```python
from build123d import *

# Parameters (mm, degrees)
BOSS_EXTRUDE1_DEPTH          = 1.5
SKETCH1_3_W                  = 3.18
SKETCH1_3_H                  = 20
CUT_EXTRUDE_THIN1_DEPTH      = 2.5
CUT_EXTRUDE_THIN1_DEPTH_BACK = 2.5
CUT_EXTRUDE1_REACH           = 5


with BuildPart() as part:
    # Sketch1 → Boss-Extrude1 (new body, symmetric)
    with BuildSketch(Plane.XY):
        Polygon((-93.914893617, 114.397705985), (-93.914893617, -65.602294015), (86.085106383, -65.602294015), (86.085106383, -25.602294015), (-3.914893617, -25.602294015), (-3.914893617, 84.397705985), (-33.914893617, 114.397705985), align=None)
    extrude(amount=BOSS_EXTRUDE1_DEPTH, both=True)

    # Sketch1_3 → Cut-Extrude-Thin1 (cut, two sides)
    with BuildSketch(Plane.XY) as cut_extrude_thin1_sk:
        with Locations((-92.414893617, 64.397705985)):
            Rectangle(SKETCH1_3_W, SKETCH1_3_H)
        with Locations((-92.414893617, 24.397705985)):
            Rectangle(SKETCH1_3_W, SKETCH1_3_H)
        with Locations((-92.414893617, -15.602294015)):
            Rectangle(SKETCH1_3_W, SKETCH1_3_H)
        with Locations((-5.414893617, 54.397705985)):
            Rectangle(SKETCH1_3_W, SKETCH1_3_H)
        with Locations((-5.414893617, 4.397705985)):
            Rectangle(SKETCH1_3_W, SKETCH1_3_H)
        with Locations((84.585106383, -45.602294015)):
            Rectangle(SKETCH1_3_W, SKETCH1_3_H)
    extrude(amount=CUT_EXTRUDE_THIN1_DEPTH, mode=Mode.SUBTRACT)
    extrude(cut_extrude_thin1_sk.sketch, amount=-CUT_EXTRUDE_THIN1_DEPTH_BACK, mode=Mode.SUBTRACT)

    # Sketch2 → Cut-Extrude1 (cut, up to next)
    with BuildSketch(Plane.XY.offset(1.5), mode=Mode.PRIVATE) as cut_extrude1_sk1:
        Polygon((-25.473348524, -46.697563546), (-7.347192784, -55.14992878), (-6.079337999, -52.431005419), (-24.205493739, -43.978640185), align=None)
    cut_extrude1_tool1 = extrude(cut_extrude1_sk1.sketch, amount=-CUT_EXTRUDE1_REACH, mode=Mode.PRIVATE) & part.part
    add(cut_extrude1_tool1.solids().sort_by_distance((-15.776343, -49.564284, 1.5))[0], mode=Mode.SUBTRACT)
    # Sketch2 → Cut-Extrude1 (cut, up to next)
    with BuildSketch(Plane.XY.offset(1.5), mode=Mode.PRIVATE) as cut_extrude1_sk2:
        Polygon((-51.39472735, -31.300092332), (-69.520883091, -22.847727097), (-70.788737876, -25.566650459), (-52.662582136, -34.019015693), align=None)
    cut_extrude1_tool2 = extrude(cut_extrude1_sk2.sketch, amount=-CUT_EXTRUDE1_REACH, mode=Mode.PRIVATE) & part.part
    add(cut_extrude1_tool2.solids().sort_by_distance((-61.091733, -28.433371, 1.5))[0], mode=Mode.SUBTRACT)


solid = part.part
```
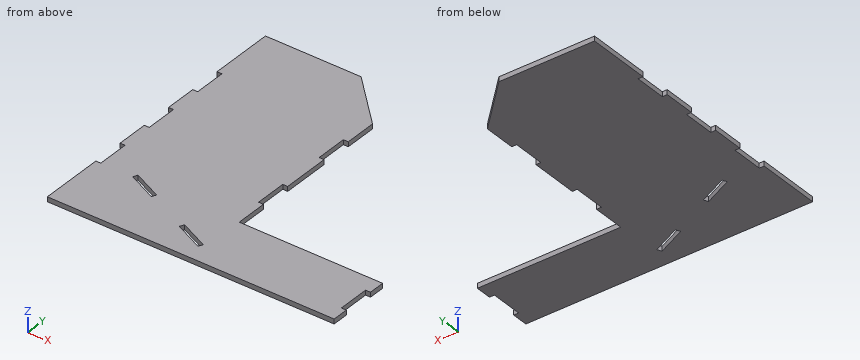
Here's how the part is built. I have some questions about the finished solid (model axes, mm). Coordinates: 2 decimals unless noted, no trailing zeros. Order: outer loops, then holes, each group sorted by start corner. A loop starts at its lowest first (then second) coordinate and runs counter-clockwise, first axis right, second up. Notation, with made-up numbers: (10, 22.25) -> (38, 22.25) arc R9 ccw to (38, 28.25) -> close; hole circle Ø2 at (-9, 11). An arc over 180 degrees is marked (long way). Return JSON: item names as keys, results as strings.
1) If we section it at D-D on x = -61.5: List the corners of the cut face in (y, z) for me.
Conclusion:
{"outline": "(-65.6, -1.5) -> (-29.9, -1.5) -> (-29.9, 1.5) -> (-65.6, 1.5) -> close; (-26.59, -1.5) -> (114.4, -1.5) -> (114.4, 1.5) -> (-26.59, 1.5) -> close"}
2) If we section it at B-B on z = -0.4: State how many separate pieces and enclosed holes the cut face has, plus the area to 3 significant figures.
Conclusion:
{"separate pieces": "1", "enclosed holes": "2", "area": "18,900 mm²"}
3) If I drill on probe 1 along X at (y, z) = (16, 0.2); probe 2 along X at (y, z) = (50, 0.9); probe 3 along Y at (x, z) = (42.5, 1.25), over which ranges is the centre line in solid material (lowest first)?
Conclusion:
{"probe 1": "x = -90.82 to -3.91", "probe 2": "x = -93.91 to -7", "probe 3": "y = -65.6 to -25.6"}
4) I'm going to push flat-ended pins straight in: P1, Ø0.9, axis at y = -14.5, z = 0, coming from the +X side; P2, Ø0.9, axis at y = 23.5, z = -0.5, coming from the -X side. Where does each tip first touch, or does it pass through?
Conclusion:
{"P1": "stops at x = -3.91", "P2": "stops at x = -90.82"}
5) If we section it at A-A on x = -18: List the corners of the cut face in (y, z) for me, plus the area to 3 significant figures.
Conclusion:
{"outline": "(-65.6, -1.5) -> (-50.18, -1.5) -> (-50.18, 1.5) -> (-65.6, 1.5) -> close; (-46.87, -1.5) -> (98.48, -1.5) -> (98.48, 1.5) -> (-46.87, 1.5) -> close", "area": "482 mm²"}
6) If we section it at C-C on y = 57: List the corners of the cut face in (x, z) for me, plus the area to 3 significant figures.
Conclusion:
{"outline": "(-90.82, -1.5) -> (-7, -1.5) -> (-7, 1.5) -> (-90.82, 1.5) -> close", "area": "251 mm²"}
